Check sheet for the drawn part. Datum: minimum x, y, z corner. Units: mm. A direction names the side the tool comes from. Round coordinates to 2 decimals unless told otherwise and drop trailing zeros. Write each loop counter-clockwise with the first axis right and the second up, starting at its lowest first coordinate (ties: lowest second). Pieces come first, ordered by that corner, then holes. Notation, with made-up numbers: M 35,15 L 59,15 A31 ccw 59,40 Z; hole C -17,63 d11. An arc over 180 degrees is marked long. Put each result on its own line as item: value.
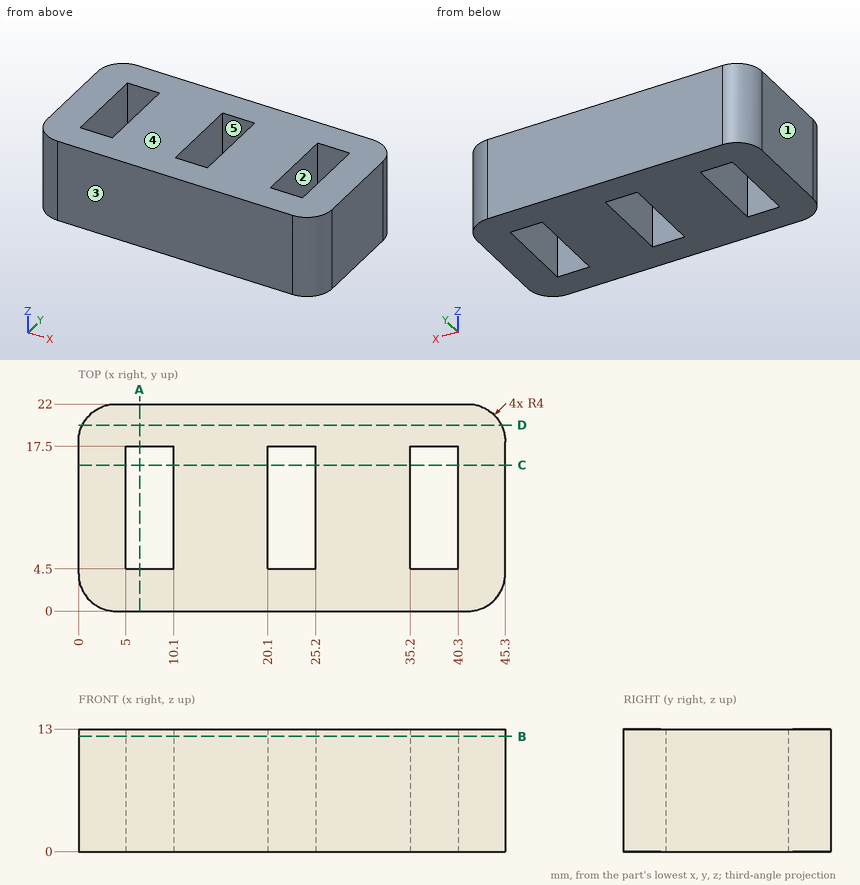
1. Access from +Z, -Z, +X, -X, +Y, -Y to the whole of each face (thin tool, end or side, straight path). Record for the marked faces 4 and 5.
Computed values:
face 4: +Z, +X, -X, +Y, -Y
face 5: +Z, -Z
2. Cross-section at C-C (y = 15.5). Enter the section's corners in (x, z).
Computed values:
outline: M 0,0 L 5,0 L 5,13 L 0,13 Z; M 10.1,0 L 20.1,0 L 20.1,13 L 10.1,13 Z; M 25.2,0 L 35.2,0 L 35.2,13 L 25.2,13 Z; M 40.3,0 L 45.3,0 L 45.3,13 L 40.3,13 Z
3. Release check for a two-part mould opening along X. For the marked faces 1, 2 and 3 record: +X half, -X half, draft (parallel to the pull), parting line (faces both ways), or undercut.
Computed values:
face 1: -X half
face 2: undercut
face 3: draft
4. Cross-section at D-D (y = 19.75). Enter the section's corners in (x, z).
Computed values:
outline: M 0.4,0 L 44.9,0 L 44.9,13 L 0.4,13 Z
5. Cross-section at B-B (z = 12.25). Enter the section's corners in (x, y).
Computed values:
outline: M 0,4 A4 ccw 4,0 L 41.3,0 A4 ccw 45.3,4 L 45.3,18 A4 ccw 41.3,22 L 4,22 A4 ccw 0,18 Z; hole M 5,4.5 L 10.1,4.5 L 10.1,17.5 L 5,17.5 Z; hole M 20.1,4.5 L 25.2,4.5 L 25.2,17.5 L 20.1,17.5 Z; hole M 35.2,4.5 L 40.3,4.5 L 40.3,17.5 L 35.2,17.5 Z
6. Cross-section at A-A (x = 6.5). Enter the section's corners in (y, z), then the cut area to 3 significant figures.
Computed values:
outline: M 0,0 L 4.5,0 L 4.5,13 L 0,13 Z; M 17.5,0 L 22,0 L 22,13 L 17.5,13 Z
area: 117 mm2
7. Scan lines: probe 1 along X at (y, z) = (16, 2); probe 2 along Y at (x, z) = (22, 3.5); probe 3 along X at (y, z) = (3.75, 7). Record each from-to range of solid material in increasing order.
Computed values:
probe 1: x = 0 to 5, 10.1 to 20.1, 25.2 to 35.2, 40.3 to 45.3
probe 2: y = 0 to 4.5, 17.5 to 22
probe 3: x = 0.01 to 45.29
